```python
from build123d import *

# Parameters (mm, degrees)
SKETCH1_R           = 2.5
BOSS_EXTRUDE1_DEPTH = 51
CUT_EXTRUDE1_DEPTH  = 15
CUT_EXTRUDE2_DEPTH  = 12.5
SKETCH4_W           = 10.949964099
SKETCH4_H           = 4
CUT_EXTRUDE3_DEPTH  = 25
SKETCH5_R           = 2
CUT_EXTRUDE4_DEPTH  = 10
FILLET4_R           = 2
FILLET5_R           = 3
FILLET6_START       = 57.196631886
FILLET6_DEPTH       = 2.760049196
FILLET6_START_2     = 53.489934113
FILLET6_2_DEPTH     = 3.979721459
FILLET6_START_3     = 57.021910195
FILLET6_3_DEPTH     = 0.447745377
FILLET6_START_4     = 1
FILLET6_4_DEPTH     = 48
FILLET6_START_5     = 46
FILLET6_5_DEPTH     = 2
FILLET6_START_6     = 2
FILLET6_6_DEPTH     = 2
SKETCH6_R           = 1.5
BOSS_EXTRUDE2_DEPTH = 5


with BuildPart() as part:
    # Sketch1 → Boss-Extrude1 (new body)
    with BuildSketch(Plane(origin=(0, 0, 0), x_dir=(1, 0, 0), z_dir=(0, 1, 0))):
        with BuildLine():
            Line((57.196631886, 9.028355512), (57.196631886, 28.639971463))
            ThreePointArc((57.196631886, 28.639971463), (52.044420209, 35.109942461), (59.956681082, 37.518663649))
            Line((59.956681082, 37.518663649), (59.956681082, 29.732723556))
            Line((59.956681082, 29.732723556), (59.956681082, 10.538718377))
            Line((59.956681082, 10.538718377), (59.030643937, 9.028355512))
            Line((59.030643937, 9.028355512), (57.196631886, 9.028355512))
        make_face()
        with Locations(Location((56.81904117, 33.625693603, 0), (0, 0, 270))):
            Circle(SKETCH1_R, mode=Mode.SUBTRACT)
    extrude(amount=BOSS_EXTRUDE1_DEPTH)

    # Sketch2 → Cut-Extrude1 (cut, symmetric)
    with BuildSketch(Plane(origin=(59.956681082, 0, 0), x_dir=(0, 0, -1), z_dir=(1, 0, 0))):
        Polygon((39.133835998, 10), (25.633835998, 10), (25.633835998, 14), (27.895137764, 14), (39.133835998, 14), align=None)
    extrude(amount=CUT_EXTRUDE1_DEPTH, both=True, mode=Mode.SUBTRACT)

    # Sketch3 → Cut-Extrude2 (cut, symmetric)
    with BuildSketch(Plane(origin=(59.956681082, 0, 0), x_dir=(0, 0, -1), z_dir=(1, 0, 0))):
        Polygon((41.711304396, 42), (27.895137764, 42), (25.633835998, 42), (25.633835998, 38), (41.711304396, 38), align=None)
    extrude(amount=CUT_EXTRUDE2_DEPTH, both=True, mode=Mode.SUBTRACT)

    # Sketch4 → Cut-Extrude3 (cut, symmetric)
    with BuildSketch(Plane(origin=(59.956681082, 0, 0), x_dir=(0, 0, -1), z_dir=(1, 0, 0))):
        with Locations((33.370119814, 2)):
            Rectangle(SKETCH4_W, SKETCH4_H)
        Polygon((38.845101863, 51), (30.056521444, 51), (27.895137764, 51), (27.895137764, 47), (27.895137764, 46), (38.845101863, 46), align=None)
    extrude(amount=CUT_EXTRUDE3_DEPTH, both=True, mode=Mode.SUBTRACT)

    # Sketch5 → Cut-Extrude4 (cut)
    with BuildSketch(Plane.ZY.offset(-57.196631886)):
        with Locations((-22.895137764, 46)):
            Circle(SKETCH5_R)
        with Locations((-14.028355512, 46)):
            Circle(SKETCH5_R)
        with Locations((-14.028355512, 6)):
            Circle(SKETCH5_R)
        with Locations((-22.895137764, 6)):
            Circle(SKETCH5_R)
    extrude(amount=-CUT_EXTRUDE4_DEPTH, mode=Mode.SUBTRACT)

    # Fillet4
    fillet4_edges = [part.edges().sort_by_distance(p)[0] for p in [
        (57.196631886, 26, -28.639971463),
    ]]
    fillet(fillet4_edges, radius=FILLET4_R)

    # Fillet5
    fillet5_edges = [part.edges().sort_by_distance(p)[0] for p in [
        (59.956681082, 7, -37.518663649),
        (59.956681082, 26, -37.518663649),
        (59.956681082, 44, -37.518663649),
    ]]
    fillet(fillet5_edges, radius=FILLET5_R)

    # Fillet6: read off the stored shape, not the designer's step
    # Fillet6 outline → Fillet6 (add)
    with BuildSketch(Plane.YZ.offset(FILLET6_START)):
        with BuildLine():
            Line((4, -27.895137764), (2, -27.895137764))
            ThreePointArc((2, -27.895137764), (3.414213563, -28.480924202), (4, -29.895137764))
            Line((4, -29.895137764), (4, -27.895137764))
        make_face()
        with BuildLine():
            Line((46, -27.895137764), (46, -29.895137764))
            ThreePointArc((46, -29.895137764), (46.585786437, -28.480924202), (48, -27.895137764))
            Line((48, -27.895137764), (46, -27.895137764))
        make_face()
        with BuildLine():
            Line((14, -25.633835998), (12, -25.633835998))
            ThreePointArc((12, -25.633835998), (13.414213562, -26.219622436), (14, -27.633835998))
            Line((14, -27.633835998), (14, -25.633835998))
        make_face()
        with BuildLine():
            ThreePointArc((10, -27.633835998), (10.585786438, -26.219622436), (12, -25.633835998))
            Line((12, -25.633835998), (10, -25.633835998))
            Line((10, -25.633835998), (10, -27.633835998))
        make_face()
        with BuildLine():
            Line((38, -25.633835998), (38, -27.633835998))
            ThreePointArc((38, -27.633835998), (38.585786438, -26.219622436), (40, -25.633835998))
            Line((40, -25.633835998), (38, -25.633835998))
        make_face()
        with BuildLine():
            Line((42, -25.633835998), (40, -25.633835998))
            ThreePointArc((40, -25.633835998), (41.414213562, -26.219622436), (42, -27.633835998))
            Line((42, -27.633835998), (42, -25.633835998))
        make_face()
    extrude(amount=FILLET6_DEPTH)

    # Fillet6 2 outline → Fillet6 2 (add)
    with BuildSketch(Plane.YZ.offset(FILLET6_START_2)):
        with BuildLine():
            Line((4, -27.895137764), (2, -27.895137764))
            ThreePointArc((2, -27.895137764), (3.414213563, -28.480924202), (4, -29.895137764))
            Line((4, -29.895137764), (4, -27.895137764))
        make_face()
        with BuildLine():
            Line((46, -27.895137764), (46, -29.895137764))
            ThreePointArc((46, -29.895137764), (46.585786437, -28.480924202), (48, -27.895137764))
            Line((48, -27.895137764), (46, -27.895137764))
        make_face()
    extrude(amount=FILLET6_2_DEPTH)

    # Fillet6 3 outline → Fillet6 3 (add)
    with BuildSketch(Plane.YZ.offset(FILLET6_START_3)):
        with BuildLine():
            Line((14, -25.633835998), (12, -25.633835998))
            ThreePointArc((12, -25.633835998), (13.414213562, -26.219622436), (14, -27.633835998))
            Line((14, -27.633835998), (14, -25.633835998))
        make_face()
        with BuildLine():
            Line((38, -25.633835998), (38, -27.633835998))
            ThreePointArc((38, -27.633835998), (38.585786438, -26.219622436), (40, -25.633835998))
            Line((40, -25.633835998), (38, -25.633835998))
        make_face()
    extrude(amount=FILLET6_3_DEPTH)

    # Fillet6 4 outline → Fillet6 4 (cut)
    with BuildSketch(Plane(origin=(0, 0, 0), x_dir=(1, 0, 0), z_dir=(0, 1, 0)).offset(FILLET6_START_4)):
        with BuildLine():
            ThreePointArc((56.880709526, 27.895137764), (56.354589633, 28.446988989), (55.660177396, 28.761843816))
            ThreePointArc((55.660177396, 28.761843816), (54.504616994, 29.193601463), (53.489934157, 29.895137813))
            Line((53.489934157, 29.895137813), (53.489934113, 27.895137764))
            Line((53.489934113, 27.895137764), (56.880709526, 27.895137764))
        make_face()
        with BuildLine():
            Line((57.196631886, 25.633835998), (57.196631886, 26.816303901))
            ThreePointArc((57.196631886, 26.816303901), (57.152463779, 27.234301039), (57.021910279, 27.633836035))
            Line((57.021910279, 27.633836035), (57.021910195, 25.633835998))
            Line((57.021910195, 25.633835998), (57.196631886, 25.633835998))
        make_face()
    extrude(amount=FILLET6_4_DEPTH, mode=Mode.SUBTRACT)

    # Fillet6 5 outline → Fillet6 5 (cut)
    with BuildSketch(Plane(origin=(0, 0, 0), x_dir=(1, 0, 0), z_dir=(0, 1, 0)).offset(FILLET6_START_5)):
        with BuildLine():
            Line((57.196631886, 27.895137764), (57.196631886, 28.639971463))
            ThreePointArc((57.196631886, 28.639971463), (56.423680429, 28.641349124), (55.660177396, 28.761843815))
            ThreePointArc((55.660177396, 28.761843815), (56.354589633, 28.446988989), (56.880709526, 27.895137764))
            Line((56.880709526, 27.895137764), (57.196631886, 27.895137764))
        make_face()
    extrude(amount=FILLET6_5_DEPTH, mode=Mode.SUBTRACT)

    # Fillet6 6 outline → Fillet6 6 (cut)
    with BuildSketch(Plane(origin=(0, 0, 0), x_dir=(1, 0, 0), z_dir=(0, 1, 0)).offset(FILLET6_START_6)):
        with BuildLine():
            Line((57.196631886, 27.895137764), (57.196631886, 28.639971463))
            ThreePointArc((57.196631886, 28.639971463), (56.423680429, 28.641349124), (55.660177396, 28.761843815))
            ThreePointArc((55.660177396, 28.761843815), (56.354589633, 28.446988989), (56.880709526, 27.895137764))
            Line((56.880709526, 27.895137764), (57.196631886, 27.895137764))
        make_face()
    extrude(amount=FILLET6_6_DEPTH, mode=Mode.SUBTRACT)

    # Sketch6 → Boss-Extrude2 (add)
    with BuildSketch(Plane(origin=(0, 30, 0), x_dir=(1, 0, 0), z_dir=(0, 1, 0))):
        with BuildLine():
            Line((57.196631886, 23.207838196), (57.196631886, 15.88036097))
            add(Edge.make_bspline(
                [(55.511713205, 17.752088745), (56.909946197, 17.31678815), (57.196631886, 15.88036097)],
                knots=[0, 0, 0, 1, 1, 1], degree=2))
            ThreePointArc((55.511713205, 17.752088745), (53.511713205, 19.752088745), (55.511713205, 21.752088745))
            add(Edge.make_bspline(
                [(55.511713205, 21.752088745), (56.732163203, 22.065636669), (57.196631886, 23.207838196)],
                knots=[0, 0, 0, 1, 1, 1], degree=2))
        make_face()
        with Locations(Location((55.511713205, 19.752088745, 0), (0, 0, 270))):
            Circle(SKETCH6_R, mode=Mode.SUBTRACT)
    extrude(amount=BOSS_EXTRUDE2_DEPTH)


solid = part.part
```
Could you check a few things on this model? Use its own coordinates, in mm. A direction names the side the tool comes from. Round coordinates to 2 decimals unless told otherwise and drop trailing zeros. Loops run counter-clockwise (first coordinate to the right, second up) from the corner with the lowest first, then second, coordinate; pieces in that order, holes last. Notation, with made-up numbers: (-37.75, -23.5) -> (6.25, -23.5) arc R22 ccw to (6.25, 6.5) -> close; hole circle Ø6 at (-29.75, 57). An arc over 180 degrees is marked (long way). Put each result on its own line as item: value.
Q1. I want a section at B-B on y = 15. Write out the boundary of the cut face in (x, z), and give its area (3 significant figures).
Checks:
outline: (55.66, -28.76) arc R5 ccw to (57.16, -38.61) arc R3 ccw to (59.96, -35.62) -> (59.96, -10.54) -> (59.03, -9.03) -> (57.2, -9.03) -> (57.2, -26.82) arc R2 cw to start; hole circle Ø5 at (56.82, -33.63)
area: 103 mm2
Q2. I want a section at A-A on y = 6. Write out the boundary of the cut face in (x, z).
Checks:
outline: (57.16, -38.61) arc R3 ccw to (59.96, -35.62) -> (59.96, -24.9) -> (57.2, -24.9) -> (57.2, -28.64) arc R5 ccw (long way) to start; (57.2, -20.9) -> (59.96, -20.9) -> (59.96, -16.03) -> (57.2, -16.03) -> close; (57.2, -12.03) -> (59.96, -12.03) -> (59.96, -10.54) -> (59.03, -9.03) -> (57.2, -9.03) -> close; hole circle Ø5 at (56.82, -33.63)
Q3. Thinking about a two-plate mould opening in Y: for faces 4 (the cylindrical face through (59.13, 26.17, -37.69)), 5 (the flat face through (57, 30, -19)), 6 (the cylindrical face through (58.469, 11.956, -25.634)), which applies, pulls with the +Y half, pulls with the -Y half, needs draft (parallel to the pull), parting line crosses it, or undercut?
Checks:
face 4: needs draft
face 5: pulls with the -Y half
face 6: undercut
Q4. I want a section at C-C on x = 58.5. Give the number of separate pieces and of enclosed holes in the cut face, and give its area (3 significant figures).
Checks:
separate pieces: 4
enclosed holes: 4
area: 1,120 mm2
Q5. Which directions (+Z, -Z, +X, -X, +Y, -Y) give clear straight access to the entire face, cutting with the end or side of a thin tool? Please do faces 1 (the flat face through (54, 42, -33)), 2 (the flat face through (54, 4, -34)), 3 (the flat face through (59, 50, -27.895)).
Checks:
face 1: -Z, +X, -X
face 2: -Z, +X, -X, -Y
face 3: -Z, +X, -X, +Y
Q6. For pin 1 Ø4.5 at (y, z) = (6, -22.9) entering from -X; pin 2 Ø4.5 at (x, z) = (56.82, -33.63) entering from +Y; pin 3 Ø4 at (x, z) = (56, -32.5) entering from -Y; pin 4 Ø1.1 at (x, z) = (54.5, -18) entering from -Y, each with a flat end and sliding along its axis, tell me the tip position at first contact or that it passes through.
Checks:
pin 1: x = 57.2
pin 2: through
pin 3: y = 4
pin 4: y = 30
Q7. I want a section at D-D on y = 43. Write out the boundary of the cut face in (x, z).
Checks:
outline: (57.16, -38.61) arc R3 ccw to (59.96, -35.62) -> (59.96, -10.54) -> (59.03, -9.03) -> (57.2, -9.03) -> (57.2, -28.64) arc R5 ccw (long way) to start; hole circle Ø5 at (56.82, -33.63)
Q8. Please list where these lines run through material, in increasing order: line 1 (Y direction, x = 53.75, z = -36.25); line 2 (Z direction, x = 54.25, y = 34); line 3 (X direction, y = 42, z = -20.25). Write a range as from..to.
Checks:
line 1: 4..10, 14..38, 42..46
line 2: -37.92..-29.34, -21.3..-20.56, -18.94..-18.2
line 3: 57.2..59.96
